The listing builds one solid part. Answer for the finished solid, in the listing's coordinates (mm). Face numbers are marked on the shaded views. A direction names the side the tool comes from. Give positions to 0.01 mm unless a question says otherwise; leave off trailing zeros. Loops run counter-clockwise (first coordinate to the right, second up) from the corner with the lowest first, then second, coordinate; pieces in that order, holes last. Notation, with made-up numbers: (27.25, 32) - (45.25, 32) arc R34 cw to (45.25, 62) - close; hole circle Ø5 at (31, 74). An arc over 180 degrees is marked (long way). Write each question's results on one line, items separated by ' | '.
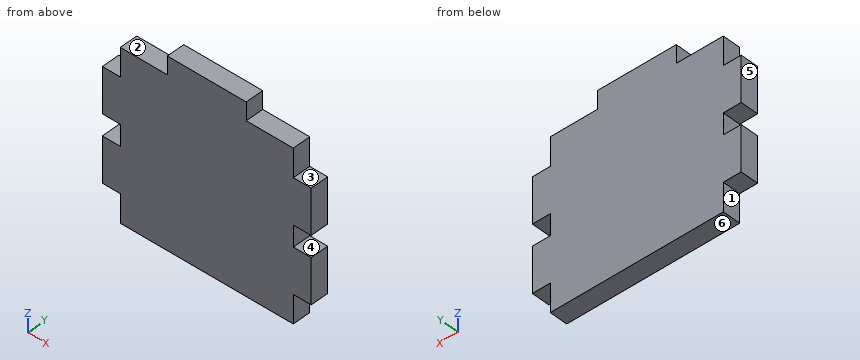
from build123d import *

# Parameters (mm, degrees)
SKETCH1_W           = 3.175
SKETCH1_H           = 8
SKETCH1_W_2         = 30.6846
SKETCH1_H_2         = 29.73
BOSS_EXTRUDE1_DEPTH = 3.175
SKETCH2_W           = 14
SKETCH2_H           = 3.175
BOSS_EXTRUDE5_DEPTH = 3.175


with BuildPart() as part:
    # Sketch1 → Boss-Extrude1 (new body)
    with BuildSketch(Plane(origin=(0, 0, 0), x_dir=(1, 0, 0), z_dir=(0, 1, 0))):
        with Locations((-16.9298, 5.865)):
            Rectangle(SKETCH1_W, SKETCH1_H)
        Rectangle(SKETCH1_W_2, SKETCH1_H_2)
        with Locations((16.9298, -5.865)):
            Rectangle(SKETCH1_W, SKETCH1_H)
        with Locations((16.9298, 5.865)):
            Rectangle(SKETCH1_W, SKETCH1_H)
        with Locations((-16.9298, -5.865)):
            Rectangle(SKETCH1_W, SKETCH1_H)
    extrude(amount=BOSS_EXTRUDE1_DEPTH)

    # Sketch2 → Boss-Extrude5 (add)
    with BuildSketch(Plane.XY.offset(14.865)):
        with Locations((0, 1.5875)):
            Rectangle(SKETCH2_W, SKETCH2_H)
    extrude(amount=BOSS_EXTRUDE5_DEPTH)


solid = part.part
Item 1: A cutting plane is placed at C-C, the plane z = 10.5. Determine the outline of the cut face in (x, y) (3 decimals), plus the area to 3 significant figures.
Values found:
outline: (-15.342, 0) - (15.342, 0) - (15.342, 3.175) - (-15.342, 3.175) - close | area: 97.4 mm²
Item 2: For the marked faces 1, 2 and 3, determine the directions among +Z, -Z, +X, -X, +Y, -Y from which every point of the face is accessible in a straight line to the end or side of a thin tool.
Values found:
face 1: -Z, -X, +Y, -Y | face 2: +Z, -X, +Y, -Y | face 3: +Z, +X, +Y, -Y
Item 3: For a pull along Z with two mould halves and no side action, classify the marked faces 4, 5 and 6 as released by +Z, released by -Z, zero draft, split by the parting line, or undercut.
Values found:
face 4: undercut | face 5: zero draft | face 6: released by -Z
Item 4: Find the intervals of material crossed by line 1 along Z through (x, y) = (12.5, 2.9) (3 decimals); line 2 along Z through (x, y) = (-15.5, 1.7) (3 decimals); line 3 along X through (y, z) = (0.5, 16.5), in increasing order. Write a range as [from, to].
Values found:
line 1: z = [-14.865, 14.865] | line 2: z = [-9.865, -1.865], [1.865, 9.865] | line 3: x = [-7, 7]
Item 5: A cutting plane is placed at B-B, the plane x = 11.5. Determine the outline of the cut face in (y, z) (3 decimals), plus the area to 3 significant figures.
Values found:
outline: (0, -14.865) - (3.175, -14.865) - (3.175, 14.865) - (0, 14.865) - close | area: 94.4 mm²
Item 6: Flat-ended cylindrical pins translate along their axes: P1, Ø1, axis at y = 1, z = 17, coming from the +X side; P2, Ø1, axis at x = -10, y = 2, coming from the +Z side (3 decimals); P3, Ø1, axis at x = -16.5, y = 2, coming from the -Z side (3 decimals). Find the tip coordinate at first contact, or state that the pin passes through.
Values found:
P1: stops at x = 7 | P2: stops at z = 14.865 | P3: stops at z = -9.865
Item 7: A cutting plane is placed at A-A, the plane y = 1.55. Determine the outline of the cut face in (x, z) (3 decimals), plus the area to 3 significant figures.
Values found:
outline: (-18.517, -9.865) - (-15.342, -9.865) - (-15.342, -14.865) - (15.342, -14.865) - (15.342, -9.865) - (18.517, -9.865) - (18.517, -1.865) - (15.342, -1.865) - (15.342, 1.865) - (18.517, 1.865) - (18.517, 9.865) - (15.342, 9.865) - (15.342, 14.865) - (7, 14.865) - (7, 18.04) - (-7, 18.04) - (-7, 14.865) - (-15.342, 14.865) - (-15.342, 9.865) - (-18.517, 9.865) - (-18.517, 1.865) - (-15.342, 1.865) - (-15.342, -1.865) - (-18.517, -1.865) - close | area: 1,060 mm²
